Work out the finished part from the listing and answer in its coordinate system (mm). Round coordinates to 2 decimals unless told otherwise and drop trailing zeros. Order: outer loops, then holes, each group sorted by start corner. A loop starts at its lowest first (then second) coordinate and runs counter-clockwise, first axis right, second up. Notation, with made-up numbers: (-0.75, 9.5) -> (37.25, 9.5) arc R28 cw to (37.25, 34.5) -> close; hole circle Ø4 at (62, -17.5). An arc over 180 degrees is marked (long way). Use a Markdown table: item, result. Add a question column.
Item 1: A flat-ended cylindrical pin translates along its axis: P1, Ø6.5, axis at x = 0, y = 0, coming from the -Z side. Find the tip coordinate at first contact, or state that the pin passes through.
Item 2: Find the intervals of material crossed by L1, parallel to Y at x = 9, z = 0.85; L2, parallel to Y at x = -32, z = 1.65; L3, parallel to X at y = 20.5, z = 2.2, in increasing order. Write a range as [from, to].
Item 3: A cutting plane is placed at D-D, the plane y = 17. Determine the outline of the cut face in (x, z).
Item 4: A cutting plane is placed at C-C, the plane x = 9. Determine the outline of the cut face in (y, z), plus the area to 3 significant figures.
Item 5: A cutting plane is placed at B-B, the plane y = 0. Determine the outline of the cut face in (x, z).
Item 6: A cutting plane is placed at A-A, the plane x = -30.5. Determine the outline of the cut face in (y, z).
from build123d import *

# Parameters (mm, degrees)
SKETCH_1_R      = 2.5
SKETCH_1_R_2    = 3.15
EXTRUDE_1_DEPTH = 4


with BuildPart() as part:
    # 草图1 → 凸台-拉伸1 (new body)
    with BuildSketch(Plane.XY):
        with BuildLine():
            ThreePointArc((-11, 10), (-3.928932188, 12.928932188), (-1, 20))
            Line((-1, 20), (-1, 39.35))
            ThreePointArc((-1, 39.35), (9, 49.35), (19, 39.35))
            Line((19, 39.35), (19, -10))
            Line((19, -10), (-32, -10))
            ThreePointArc((-32, -10), (-42, 0), (-32, 10))
            Line((-32, 10), (-11, 10))
        make_face()
        with Locations((-32, 0)):
            Circle(SKETCH_1_R, mode=Mode.SUBTRACT)
        with Locations((9, 39.35)):
            Circle(SKETCH_1_R_2, mode=Mode.SUBTRACT)
        Circle(SKETCH_1_R, mode=Mode.SUBTRACT)
    extrude(amount=EXTRUDE_1_DEPTH)


solid = part.part
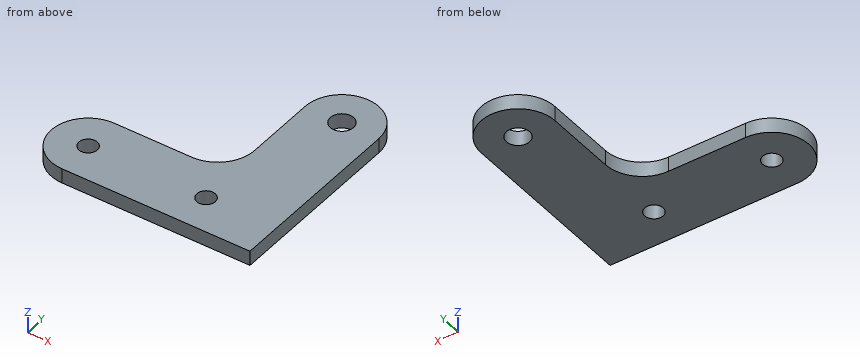
Reported:
| question | item | result |
|---|---|---|
| 1 | P1 | z = 0 |
| 2 | L1 | [-10, 36.2], [42.5, 49.35] |
| 2 | L2 | [-10, -2.5], [2.5, 10] |
| 2 | L3 | [-1, 19] |
| 3 | outline | (-1.46, 0) -> (19, 0) -> (19, 4) -> (-1.46, 4) -> close |
| 4 | outline | (-10, 0) -> (36.2, 0) -> (36.2, 4) -> (-10, 4) -> close; (42.5, 0) -> (49.35, 0) -> (49.35, 4) -> (42.5, 4) -> close |
| 4 | area | 212 mm² |
| 5 | outline | (-42, 0) -> (-34.5, 0) -> (-34.5, 4) -> (-42, 4) -> close; (-29.5, 0) -> (-2.5, 0) -> (-2.5, 4) -> (-29.5, 4) -> close; (2.5, 0) -> (19, 0) -> (19, 4) -> (2.5, 4) -> close |
| 6 | outline | (-10, 0) -> (-2, 0) -> (-2, 4) -> (-10, 4) -> close; (2, 0) -> (10, 0) -> (10, 4) -> (2, 4) -> close |
